CAD build for the part. Positions are in the model's coordinates, mm. Face numbers are marked on the shaded views. Coordinates: 2 decimals unless noted, no trailing zeros. Order: outer loops, then holes, each group sorted by start corner. A loop starts at its lowest first (then second) coordinate and runs counter-clockwise, first axis right, second up. Notation, with made-up numbers: (-21.5, 66) - (33.5, 66) arc R18 ccw to (33.5, 100) - close; hole circle Ø5 at (-39, -37). An arc over 180 degrees is marked (long way). Use one line per item in the form item = value.
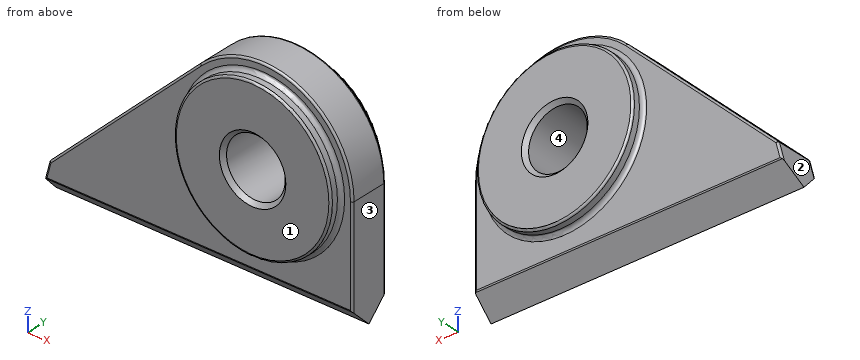
```python
from build123d import *

# Parameters (mm, degrees)
F0_R     = 20
F1_DEPTH = 5
F0_R_2   = 7.5
F2_DEPTH = 8
F3_R     = 1
F4_SIZE  = 1
F6_DEPTH = 80.001
F7_R     = 0.5


with BuildPart() as f1:
    # F0 (on Front) → F1 (new body, symmetric)
    with BuildSketch(Plane.XZ):
        with BuildLine():
            Line((23, -30), (23, 0))
            ThreePointArc((23, 0), (8.9768012825, 21.175859811), (-15.9927859769, 16.5296943922))
            Line((-15.9927859769, 16.5296943922), (-54.5205736666, -20.7466549501))
            Line((-54.5205736666, -20.7466549501), (-57, -30))
            Line((-57, -30), (23, -30))
        make_face()
        Circle(F0_R, mode=Mode.SUBTRACT)
    extrude(amount=F1_DEPTH, both=True)

    # F0 (on Front) → F2 (join, symmetric)
    with BuildSketch(Plane.XZ):
        Circle(F0_R)
        Circle(F0_R_2, mode=Mode.SUBTRACT)
    extrude(amount=F2_DEPTH, both=True)

    # F3
    f3_edges = [f1.edges().sort_by_distance(p)[0] for p in [
        (-20, -5, 0),
        (-20, 5, 0),
    ]]
    fillet(f3_edges, radius=F3_R)

    # F4
    f4_edges = [f1.edges().sort_by_distance(p)[0] for p in [
        (-7.5, -8, 0),
        (7.5, 0, 0),
        (-7.5, 8, 0),
    ]]
    chamfer(f4_edges, length=F4_SIZE)

    # F5 (on face) → F6 (cut, through all)
    with BuildSketch(Plane.YZ.offset(23)):
        Polygon((5, -25), (0, -30), (-5, -25), (-8.4046628326, -25), (-8.4046628326, -34.2726558447), (0, -34.2726558447), (8.4046628326, -34.2726558447), (8.4046628326, -25), align=None)
    extrude(amount=-F6_DEPTH, mode=Mode.SUBTRACT)

    # F7
    f7_edges = [f1.edges().sort_by_distance(p)[0] for p in [
        (-20, -8, 0),
        (-20, 8, 0),
        (-16.330127, 5, -25),
        (-55.090414, 5, -22.873327),
        (-35.25668, 5, -2.10848),
        (-16.330127, -5, -25),
        (-55.090414, -5, -22.873327),
        (23, -5, -12.5),
        (-54.520574, 0, -20.746655),
    ]]
    fillet(f7_edges, radius=F7_R)


solid = f1.part
```
Item 1: Drop flat-ended pins along their axis: pin 1 (14 mm diameter, centred on x = -26, z = -5.5, fed in from -Y); pin 2 (1 mm diameter, centred on x = -30.5, y = 1.5, fed in from -Z); pin 3 (12 mm diameter, centred on x = -48.5, z = -10.5, fed in from -Y). Give the stop position or say it passes through.
Derived:
pin_1 = -7.99
pin_2 = -29
pin_3 = -5
Item 2: Drill centre lines: line 1 (X direction, y = -4.5, z = -6.5); line 2 (Y direction, x = -21.5, z = -9.5); line 3 (Z direction, x = -3.5, y = 6). Where is each one in solid material? Low to high. Write a range as [from, to].
Derived:
line_1 = [-39.8, -3.74], [3.74, 23]
line_2 = [-5, 5]
line_3 = [-19.69, -6.63], [6.63, 19.69]
Item 3: Cut at A-A, the plane y = 2.5. Write the cut outline in (x, z).
Derived:
outline = (-56.33, -27.5) - (23, -27.5) - (23, 0) arc R23 ccw to (-15.99, 16.53) - (-54.42, -20.65) arc R0.5 ccw to (-54.56, -20.88) - close; hole circle Ø15 at (0, 0)
Item 4: Two-plate mould, pull along X, no slides. Class the marked faces 1, 2, 3 and 4: +X half, -X half, draft (parallel to the pull), parting line (faces both ways), or undercut.
Derived:
face_1 = draft
face_2 = -X half
face_3 = +X half
face_4 = undercut
